Answer from the drawing. Dimensions are ordinates in mm from the lowest x, y and z of the part. A direction names the side the tool comes from. Give positions to 0.01 mm unless a question says otherwise; leave off trailing zeros. Order: outer loops, then holes, each group sorted by start corner. A loop starts at its lowest first (then second) coordinate and runs counter-clockwise, first axis right, second up. Notation, with made-up numbers: (63.5, -10.75) - (75.5, -10.75) arc R22 ccw to (75.5, 14.25) - close; hole circle Ø10 at (80.25, 71.5). An arc over 180 degrees is marked (long way). Write each question's results on one line, items separated by ' | '.
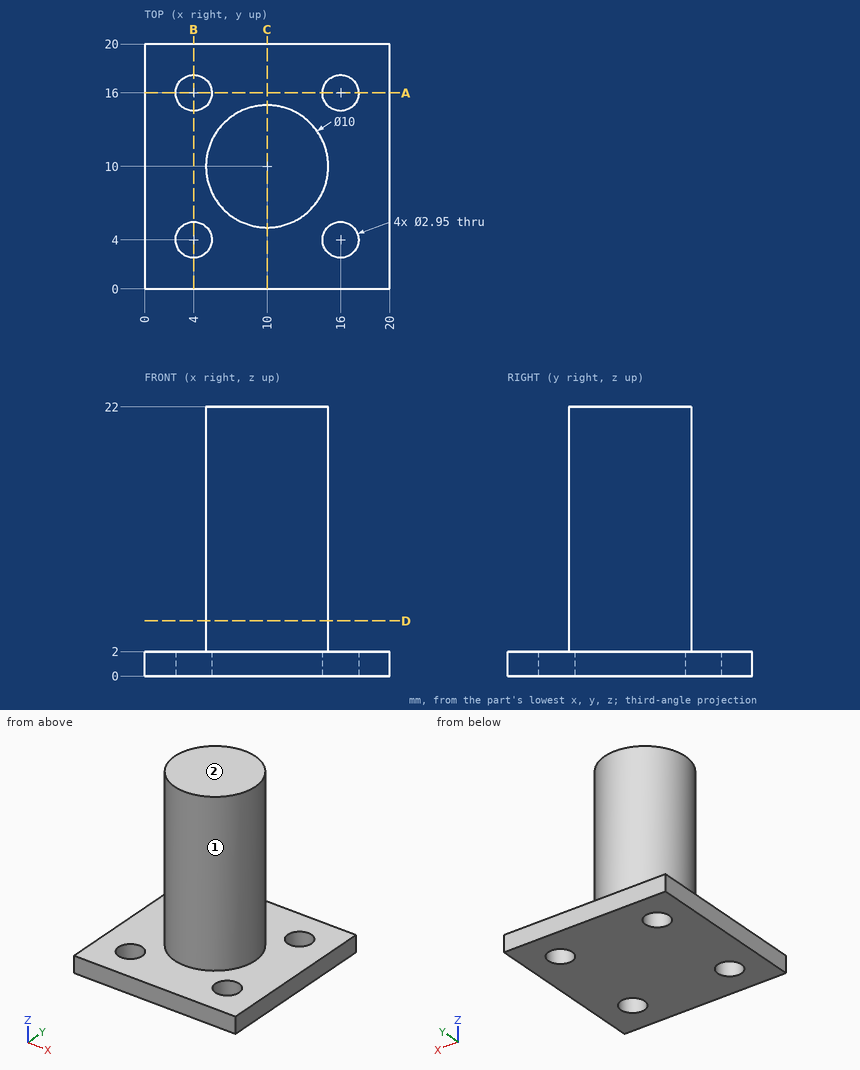
1. A cutting plane is placed at D-D, the plane z = 4.5. Write down the section's boundary in (x, y).
Answer list:
outline: circle Ø10 at (10, 10)
2. A cutting plane is placed at A-A, the plane y = 16. Write down the section's boundary in (x, z) (3 decimals), then the cut area to 3 significant figures.
Answer list:
outline: (0, 0) - (2.525, 0) - (2.525, 2) - (0, 2) - close; (5.475, 0) - (14.525, 0) - (14.525, 2) - (5.475, 2) - close; (17.475, 0) - (20, 0) - (20, 2) - (17.475, 2) - close | area: 28.2 mm^2
3. Straight lines are drawn through the part: line 1 (Y direction, x = 4, z = 1.35) (3 decimals); line 2 (Y direction, x = 2.75, z = 1). For each, find the intervals that lie inside material, in ascending order. Write a range as [from, to].
Answer list:
line 1: [0, 2.525], [5.475, 14.525], [17.475, 20] | line 2: [0, 3.22], [4.78, 15.22], [16.78, 20]
4. A cutting plane is placed at C-C, the plane x = 10. Write down the section's boundary in (y, z).
Answer list:
outline: (0, 0) - (20, 0) - (20, 2) - (15, 2) - (15, 22) - (5, 22) - (5, 2) - (0, 2) - close
5. A tool of negligible diameter and unlimited length cuts with its end or side. For the marked faces 1 and 2, from which of +Z, -Z, +X, -X, +Y, -Y can it reach the whole face along a straight path? Write none if from no direction.
Answer list:
face 1: +Z | face 2: +Z, +X, -X, +Y, -Y
6. Given P1, Ø4.5, axis at x = 4, y = 4, coming from the +Z side; P2, Ø12, axis at x = 4.5, y = 5.5, coming from the +Z side; P3, Ø6, axis at x = 11, z = 19.5, coming from the -Y side; P4, Ø6, axis at x = 12, z = 8.5, coming from the +Y side, each flat-ended and moving along its own axis, determine where each tip first touches the part or whether it passes through.
Answer list:
P1: z = 2 | P2: z = 22 | P3: y = 5 | P4: y = 15
